Could you check a few things on this model? Use its own coordinates, in mm. A direction names the side the tool comes from. Round coordinates to 2 decimals unless told otherwise and drop trailing zeros. Write each loop counter-clockwise with the first axis right and the second up, starting at its lowest first coordinate (ties: lowest second). Pieces come first, ordered by that corner, then holes. Notation, with made-up numbers: (57.25, 19) - (95.25, 19) arc R18 cw to (95.25, 47) - close; hole circle Ø11 at (14, 82.5). An arc over 180 degrees is marked (long way). Put each result on its own line as item: value.
from build123d import *

# Parameters (mm, degrees)
SKETCH1_R           = 4.6
BOSS_EXTRUDE1_DEPTH = 0.75
SKETCH2_R           = 4
BOSS_EXTRUDE2_DEPTH = 1.75
SKETCH3_R           = 2.5
CUT_EXTRUDE1_DEPTH  = 3.5
FILLET1_R           = 0.06


with BuildPart() as part:
    # Sketch1 → Boss-Extrude1 (new body)
    with BuildSketch(Plane.XY):
        Circle(SKETCH1_R)
    extrude(amount=BOSS_EXTRUDE1_DEPTH)

    # Sketch2 → Boss-Extrude2 (add)
    with BuildSketch(Plane.XY.offset(0.75)):
        Circle(SKETCH2_R)
    extrude(amount=BOSS_EXTRUDE2_DEPTH)

    # Sketch3 → Cut-Extrude1 (cut, through all)
    with BuildSketch(Plane.XY.offset(2.5)):
        with Locations((-0.193142298, 0)):
            Circle(SKETCH3_R)
    extrude(amount=-CUT_EXTRUDE1_DEPTH, mode=Mode.SUBTRACT)

    # Fillet1
    fillet1_edges = [part.edges().sort_by_distance(p)[0] for p in [
        (-4.6, 0, 0),
        (-4.6, 0, 0.75),
        (-4, 0, 2.5),
    ]]
    fillet(fillet1_edges, radius=FILLET1_R)


solid = part.part
(1) Imagine slicing it at A-A, the plane y = 0. List the corners of the cut face in (x, z) for me, then the cut area to 3 significant figures.
Values found:
outline: (-4.6, 0.06) arc R0.06 ccw to (-4.54, 0) - (-2.69, 0) - (-2.69, 2.5) - (-3.94, 2.5) arc R0.06 ccw to (-4, 2.44) - (-4, 0.75) - (-4.54, 0.75) arc R0.06 ccw to (-4.6, 0.69) - close; (2.31, 0) - (4.54, 0) arc R0.06 ccw to (4.6, 0.06) - (4.6, 0.69) arc R0.06 ccw to (4.54, 0.75) - (4, 0.75) - (4, 2.44) arc R0.06 ccw to (3.94, 2.5) - (2.31, 2.5) - close
area: 8.40 mm^2
(2) I'm going to push a flat-ended pin straight in: pin 1 (1 mm diameter, centred on y = -1, z = 2, fed in from +X). Where does the tip first touch, or does it pass through?
Values found:
pin 1: stops at x = 3.97
(3) Imagine slicing it at D-D, the plane z = 0.5. List the corners of the cut face in (x, y) for me, then the cut area to 3 significant figures.
Values found:
outline: circle Ø9.2 at (0, 0); hole circle Ø5 at (-0.19, 0)
area: 46.8 mm^2
(4) Imagine slicing it at B-B, the plane z = 2. List the corners of the cut face in (x, y) for me.
Values found:
outline: circle Ø8 at (0, 0); hole circle Ø5 at (-0.19, 0)
(5) If we mould it in two halves opening along Z, with no side actions, what happens to faces 1 (the face through (-3.65, -2.8, 0.37)), 2 (the face through (3, -3, 0.75)), 3 (the face through (2, -2, 0))? For each: pulls with the +Z half, pulls with the -Z half, needs draft (parallel to the pull), parting line crosses it, or undercut.
Values found:
face 1: needs draft
face 2: pulls with the +Z half
face 3: pulls with the -Z half
(6) For faces 4 (the face through (2, -2, 2.5)), 5 (the face through (-0.867, -3.905, 1.583)), which set-ups out of +Z, -Z, +X, -X, +Y, -Y let a thin tool reach every point of the face, with its end or its side?
Values found:
face 4: +Z, +X, -X, +Y, -Y
face 5: +Z
(7) Please list where these lines run through material, in increasing order: probe 1 along Y at (x, z) = (-0.75, 1.5); probe 2 along Y at (x, z) = (0, 1.4); probe 3 along X at (y, z) = (0.25, 2.25). Write a range as from..to.
Values found:
probe 1: y = -3.93..-2.44, 2.44..3.93
probe 2: y = -4..-2.49, 2.49..4
probe 3: x = -3.99..-2.68, 2.29..3.99
(8) Imagine slicing it at C-C, the plane x = 0. List the corners of the cut face in (y, z) for me, then the cut area to 3 significant figures.
Values found:
outline: (-4.6, 0.06) arc R0.06 ccw to (-4.54, 0) - (-2.49, 0) - (-2.49, 2.5) - (-3.94, 2.5) arc R0.06 ccw to (-4, 2.44) - (-4, 0.75) - (-4.54, 0.75) arc R0.06 ccw to (-4.6, 0.69) - close; (2.49, 0) - (4.54, 0) arc R0.06 ccw to (4.6, 0.06) - (4.6, 0.69) arc R0.06 ccw to (4.54, 0.75) - (4, 0.75) - (4, 2.44) arc R0.06 ccw to (3.94, 2.5) - (2.49, 2.5) - close
area: 8.43 mm^2
